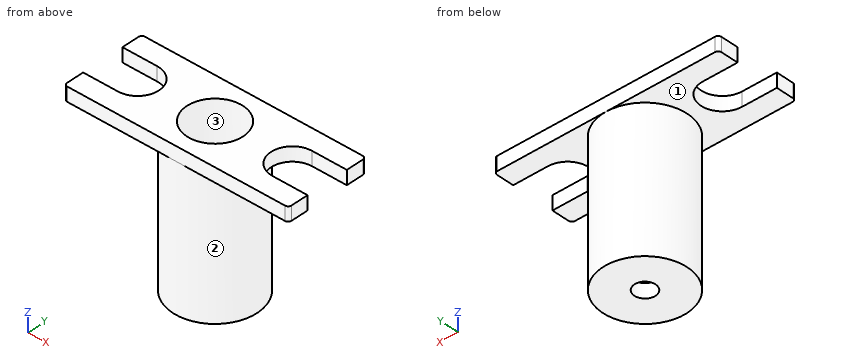
from build123d import *

# Parameters (mm, degrees)
F0_R     = 19.05
F1_DEPTH = 69.85
F2_R     = 12.7
F3_DEPTH = 63.5
F4_R     = 4.7625
F5_DEPTH = 69.851
F7_DEPTH = 6.35
F8_ANGLE = 90


with BuildPart() as f1:
    # F0 (on Top) → F1 (new body)
    with BuildSketch(Plane.XY):
        Circle(F0_R)
    extrude(amount=F1_DEPTH)

    # F2 (on face) → F3 (cut)
    with BuildSketch(Plane.XY.offset(69.85)):
        Circle(F2_R)
    extrude(amount=-F3_DEPTH, mode=Mode.SUBTRACT)

    # F4 (on face) → F5 (cut, through all)
    with BuildSketch(Plane(origin=(0, 0, 0), x_dir=(1, 0, 0), z_dir=(0, 0, -1))):
        Circle(F4_R)
    extrude(amount=-F5_DEPTH, mode=Mode.SUBTRACT)

    # F6 (on face) → F7 (join)
    with BuildSketch(Plane.XY.offset(69.85)):
        with BuildLine():
            Line((9.652, -50.8), (17.526, -50.8))
            ThreePointArc((17.526, -50.8), (18.6036307345, -50.3536307345), (19.05, -49.276))
            Line((19.05, -49.276), (19.05, 0))
            ThreePointArc((19.05, 0), (7.1e-09, -19.05), (-19.05, -1.43e-08))
            Line((-19.05, -1.43e-08), (-19.05, -49.276))
            ThreePointArc((-19.05, -49.276), (-18.6036307345, -50.3536307345), (-17.526, -50.8))
            Line((-17.526, -50.8), (-9.652, -50.8))
            Line((-9.652, -50.8), (-9.652, -35.052))
            ThreePointArc((-9.652, -35.052), (0, -25.4), (9.652, -35.052))
            Line((9.652, -35.052), (9.652, -50.8))
        make_face()
        with BuildLine():
            ThreePointArc((-19.05, -1.43e-08), (-7.1e-09, 19.05), (19.05, 0))
            Line((19.05, 0), (19.05, 49.276))
            ThreePointArc((19.05, 49.276), (18.6036307345, 50.3536307345), (17.526, 50.8))
            Line((17.526, 50.8), (9.652, 50.8))
            Line((9.652, 50.8), (9.652, 35.052))
            ThreePointArc((9.652, 35.052), (0, 25.4), (-9.652, 35.052))
            Line((-9.652, 35.052), (-9.652, 50.8))
            Line((-9.652, 50.8), (-17.526, 50.8))
            ThreePointArc((-17.526, 50.8), (-18.6036307345, 50.3536307345), (-19.05, 49.276))
            Line((-19.05, 49.276), (-19.05, -1.43e-08))
        make_face()
    extrude(amount=-F7_DEPTH)


with BuildPart() as f1_1:
    # F8: moved
    add(f1.part.rotate(Axis((0, 0, 69.85), (0, 0, 1)), F8_ANGLE))


solid = f1_1.part
CAD build for the part. Positions are in the model's coordinates, mm. Face numbers are marked on the shaded views. Give positions to 0.01 mm unless a question says otherwise; leave off trailing zeros. Loops run counter-clockwise (first coordinate to the right, second up) from the corner with the lowest first, then second, coordinate; pieces in that order, holes last. Notation, with made-up numbers: M 2,-33 L 18,-33 A32 cw 18,-4 Z; hole C 73,53 d6. An arc over 180 degrees is marked long. One line per question, with ' | ' between items. Start each with the question number.
1. Saw through at D-D on z = 23. Give the cut face in (x, y), plus the area to 3 significant figures.
2. Two-plate mould, pull along Y, no slides. Class the marked faces 1, 2 and 3: pulls with the +Y half, pulls with the -Y half, needs draft (parallel to the pull), parting line crosses it, or undercut.
3. Saw through at B-B on x = -38. Give the cut face in (y, z), plus the area to 3 significant figures.
4. Saw through at C-C on y = -15. Give the cut face in (x, z), plus the area to 3 significant figures.
5. Probe L1, parallel to X at y = 0, z = 48.5; L2, parallel to X at y = 0, z = 5; L3, parallel to Z at x = 33, y = -9.5. List the from-to ranges inside material, lowest first. Write a range as from..to.
6. Flat gauge pins, fed straight in: pin 1 (8 mm diameter, centred on y = -13.5, z = 47.5, fed in from +X); pin 2 (12.5 mm diameter, centred on x = 0, y = 0, fed in from +Z); pin 3 (3 mm diameter, centred on y = 14, z = 27.5, fed in from -X). Where does each tip first touch, or does it go through?
7. Saw through at A-A on y = 0. Give the cut face in (x, z), plus the area to 3 significant figures.
Result sheet:
1) outline: C 0,0 d38.1; hole C 0,0 d25.4 | area: 633 mm^2
2) face 1: needs draft | face 2: parting line crosses it | face 3: undercut
3) outline: M -19.05,63.5 L -9.65,63.5 L -9.65,69.85 L -19.05,69.85 Z; M 9.65,63.5 L 19.05,63.5 L 19.05,69.85 L 9.65,69.85 Z | area: 119 mm^2
4) outline: M -50.8,63.5 L -11.74,63.5 L -11.74,0 L 11.74,0 L 11.74,63.5 L 50.8,63.5 L 50.8,69.85 L -50.8,69.85 Z | area: 2,140 mm^2
5) L1: x = -19.05..-12.7, 12.7..19.05 | L2: x = -19.05..-4.76, 4.76..19.05 | L3: z = 63.5..69.85
6) pin 1: stops at x = 16.51 | pin 2: stops at z = 6.35 | pin 3: stops at x = -14.38
7) outline: M -25.4,63.5 L -19.05,63.5 L -19.05,0 L -4.76,0 L -4.76,6.35 L -12.7,6.35 L -12.7,69.85 L -25.4,69.85 Z; M 4.76,0 L 19.05,0 L 19.05,63.5 L 25.4,63.5 L 25.4,69.85 L 12.7,69.85 L 12.7,6.35 L 4.76,6.35 Z | area: 1,070 mm^2
